Read the model definition and answer for the solid it produces. Units are mm, in the model's axes. Face numbers are marked on the shaded views. A direction names the side the tool comes from. Coordinates: 2 decimals unless noted, no trailing zeros. Order: outer loops, then holes, each group sorted by start corner. A loop starts at its lowest first (then second) coordinate and runs counter-clockwise, first axis right, second up. Notation, with made-up numbers: (34, -13) -> (54, -13) arc R30 ccw to (54, 16) -> close; hole circle Ø4 at (28, -20.75). An arc over 180 degrees is marked (long way). Answer in a Markdown table with one row per item.
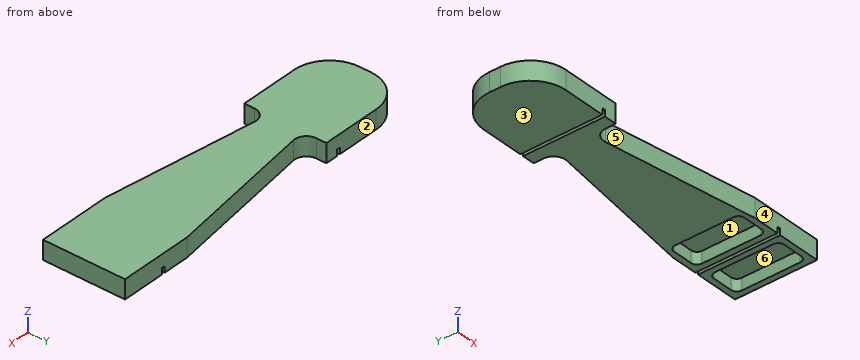
from build123d import *

# Parameters (mm, degrees)
F0_W      = 179.2732
F0_H      = 31.5976
F1_DEPTH  = 22.0853
F2_W      = 1.7526
F2_H      = 3.3528
F3_DEPTH  = 44.1716
F4_W      = 179.2732
F4_H      = 21.4376
F5_DEPTH  = 44.1716
F7_DEPTH  = 10.161
F9_DEPTH  = 6.35
F11_DEPTH = 10.161


with BuildPart() as f1:
    # F0 (on Front) → F1 (new body, symmetric)
    with BuildSketch(Plane.XZ):
        with Locations((89.6366, 15.7988)):
            Rectangle(F0_W, F0_H)
    extrude(amount=F1_DEPTH, both=True)

    # F2 (on face) → F3 (cut, through all)
    with BuildSketch(Plane.XZ.offset(22.0853)):
        with Locations((43.1419, 1.6764)):
            Rectangle(F2_W, F2_H)
        with Locations((154.9019, 1.6764)):
            Rectangle(F2_W, F2_H)
    extrude(amount=-F3_DEPTH, mode=Mode.SUBTRACT)

    # F4 (on face) → F5 (cut, through all)
    with BuildSketch(Plane.XZ.offset(22.0853)):
        with Locations((89.6366, 20.8788)):
            Rectangle(F4_W, F4_H)
    extrude(amount=-F5_DEPTH, mode=Mode.SUBTRACT)

    # F6 (on face) → F7 (cut, through all)
    with BuildSketch(Plane.XY.offset(10.16)):
        with BuildLine():
            Line((58.048026, 10.420732), (139.7, 22.0853))
            Line((139.7, 22.0853), (50.8, 22.0853))
            Line((50.8, 22.0853), (50.8, 16.706912))
            ThreePointArc((50.8, 16.706912), (52.989469, 11.909779), (58.048026, 10.420732))
        make_face()
        with BuildLine():
            Line((139.7, -22.0853), (58.048026, -10.420732))
            ThreePointArc((58.048026, -10.420732), (52.989469, -11.909779), (50.8, -16.706912))
            Line((50.8, -16.706912), (50.8, -22.0853))
            Line((50.8, -22.0853), (139.7, -22.0853))
        make_face()
    extrude(amount=-F7_DEPTH, mode=Mode.SUBTRACT)

    # F8 (on face) → F9 (cut)
    with BuildSketch(Plane(origin=(0, 0, 0), x_dir=(1, 0, 0), z_dir=(0, 0, -1))):
        with BuildLine():
            Line((172.9232, 18.9103), (162.1282, 18.9103))
            ThreePointArc((162.1282, 18.9103), (159.883136, 17.980364), (158.9532, 15.7353))
            Line((158.9532, 15.7353), (158.9532, -15.7353))
            ThreePointArc((158.9532, -15.7353), (159.883136, -17.980364), (162.1282, -18.9103))
            Line((162.1282, -18.9103), (172.9232, -18.9103))
            ThreePointArc((172.9232, -18.9103), (175.168264, -17.980364), (176.0982, -15.7353))
            Line((176.0982, -15.7353), (176.0982, 15.7353))
            ThreePointArc((176.0982, 15.7353), (175.168264, 17.980364), (172.9232, 18.9103))
        make_face()
        with BuildLine():
            Line((147.5232, 18.9103), (136.7282, 18.9103))
            ThreePointArc((136.7282, 18.9103), (134.483136, 17.980364), (133.5532, 15.7353))
            Line((133.5532, 15.7353), (133.5532, -15.7353))
            ThreePointArc((133.5532, -15.7353), (134.483136, -17.980364), (136.7282, -18.9103))
            Line((136.7282, -18.9103), (147.5232, -18.9103))
            ThreePointArc((147.5232, -18.9103), (149.768264, -17.980364), (150.6982, -15.7353))
            Line((150.6982, -15.7353), (150.6982, 15.7353))
            ThreePointArc((150.6982, 15.7353), (149.768264, 17.980364), (147.5232, 18.9103))
        make_face()
    extrude(amount=-F9_DEPTH, mode=Mode.SUBTRACT)

    # F10 (on face) → F11 (cut, through all)
    with BuildSketch(Plane.XY.offset(10.16)):
        with BuildLine():
            ThreePointArc((0, 3.0353), (5.579616, 16.505684), (19.05, 22.0853))
            Line((19.05, 22.0853), (0, 22.0853))
            Line((0, 22.0853), (0, 3.0353))
        make_face()
        with BuildLine():
            ThreePointArc((19.05, -22.0853), (5.579616, -16.505684), (0, -3.0353))
            Line((0, -3.0353), (0, -22.0853))
            Line((0, -22.0853), (19.05, -22.0853))
        make_face()
    extrude(amount=-F11_DEPTH, mode=Mode.SUBTRACT)


solid = f1.part
Q1. For the marked faces 4, 5 and 6, determine the directions among +Z, -Z, +X, -X, +Y, -Y from which every point of the face is accessible in a straight line to the end or side of a thin tool.
Outcome:
| item | result |
|---|---|
| face 4 | +Z, -Z, +X, -X, -Y |
| face 5 | +Z, -Z, -Y |
| face 6 | -Z |
Q2. Given pin 1 (0.5 mm diameter, centred on x = 155, y = 10.5, fed in from -Z); pin 2 (2.5 mm diameter, centred on y = 6, z = 1.5, fed in from -X); pin 3 (8.5 mm diameter, centred on x = 139.5, y = -4.5, fed in from -Z), each flat-ended and moving along its own axis, determine where each tip first touches the part or whether it passes through.
Outcome:
| item | result |
|---|---|
| pin 1 | z = 3.35 |
| pin 2 | x = 0.08 |
| pin 3 | z = 6.35 |
Q3. For a pull along Y with two mould halves and no side action, classify the marked faces 1, 2 and 3 as pulls with the +Y half, pulls with the -Y half, needs draft (parallel to the pull), parting line crosses it, or undercut.
Outcome:
| item | result |
|---|---|
| face 1 | undercut |
| face 2 | pulls with the +Y half |
| face 3 | needs draft |
Q4. The part is cut by section D-D (y = -6). Write down the section's boundary in (x, z), then the cut area to 3 significant figures.
Outcome:
| item | result |
|---|---|
| outline | (0.23, 0) -> (42.27, 0) -> (42.27, 3.35) -> (44.02, 3.35) -> (44.02, 0) -> (133.55, 0) -> (133.55, 6.35) -> (150.7, 6.35) -> (150.7, 0) -> (154.03, 0) -> (154.03, 3.35) -> (155.78, 3.35) -> (155.78, 0) -> (158.95, 0) -> (158.95, 6.35) -> (176.1, 6.35) -> (176.1, 0) -> (179.27, 0) -> (179.27, 10.16) -> (0.23, 10.16) -> close |
| area | 1,590 mm² |
Q5. The part is cut by section A-A (z = 8.5). Write down the section's boundary in (x, y).
Outcome:
| item | result |
|---|---|
| outline | (0, -3.04) arc R19.05 ccw to (19.05, -22.09) -> (50.8, -22.09) -> (50.8, -16.71) arc R6.35 cw to (58.05, -10.42) -> (139.7, -22.09) -> (179.27, -22.09) -> (179.27, 22.09) -> (139.7, 22.09) -> (58.05, 10.42) arc R6.35 cw to (50.8, 16.71) -> (50.8, 22.09) -> (19.05, 22.09) arc R19.05 ccw to (0, 3.04) -> close |
Q6. The part is cut by section B-B (y = -13.5). Write down the section's boundary in (x, z).
Outcome:
| item | result |
|---|---|
| outline | (3.13, 0) -> (42.27, 0) -> (42.27, 3.35) -> (44.02, 3.35) -> (44.02, 0) -> (51.67, 0) -> (51.67, 10.16) -> (3.13, 10.16) -> close; (79.6, 0) -> (133.55, 0) -> (133.55, 6.35) -> (150.7, 6.35) -> (150.7, 0) -> (154.03, 0) -> (154.03, 3.35) -> (155.78, 3.35) -> (155.78, 0) -> (158.95, 0) -> (158.95, 6.35) -> (176.1, 6.35) -> (176.1, 0) -> (179.27, 0) -> (179.27, 10.16) -> (79.6, 10.16) -> close |
Q7. The part is cut by section C-C (x = 141.5). Write down the section's boundary in (y, z), then the cut area to 3 significant figures.
Outcome:
| item | result |
|---|---|
| outline | (-22.09, 0) -> (-18.91, 0) -> (-18.91, 6.35) -> (18.91, 6.35) -> (18.91, 0) -> (22.09, 0) -> (22.09, 10.16) -> (-22.09, 10.16) -> close |
| area | 209 mm² |
Q8. Consider line 1 (X direction, y = 2, z = 5.25); line 2 (X direction, y = 7.5, z = 0.5); line 3 (X direction, y = -1.5, z = 2.75). Determine where each line is inside the solid, lowest interval first.
Outcome:
| item | result |
|---|---|
| line 1 | 0 to 133.55, 150.7 to 158.95, 176.1 to 179.27 |
| line 2 | 0.53 to 42.27, 44.02 to 133.55, 150.7 to 154.03, 155.78 to 158.95, 176.1 to 179.27 |
| line 3 | 0 to 42.27, 44.02 to 133.55, 150.7 to 154.03, 155.78 to 158.95, 176.1 to 179.27 |
